Autodesk Inventor part; units mm, degrees
ref_plane "YZ Plane" through (0, 0, 0) normal (1, 0, 0) x (0, 1, 0)
ref_plane "XZ Plane" through (0, 0, 0) normal (0, 1, 0) x (-1, 0, 0)
ref_plane "XY Plane" through (0, 0, 0) normal (0, 0, 1) x (1, 0, 0)
sketch "Sketch1" plane through (0, 0, 0) normal (0, 1, 0) x (-1, 0, 0)
  circle A0 centre (0, 0) radius 63.5
  dimension "d0" = 127
extrude "Extrusion1" add sketch "Sketch1" along normal blind 10
sketch "Sketch2" plane through (0, 0, 0) normal (0, -1, 0) x (1, 0, 0)
  circle A0 centre (0, -44.45) radius 5
  line L0 (0, 0) -> (0, -44.45)
  dimension "d3" = 44.45
  dimension "d4" = 10
extrude "Extrusion2" add sketch "Sketch2" along normal blind 20
sketch "Sketch3" plane through (0, -20, -44.45) normal (0, -1, 0) x (1, 0, 0)
  circle A0 centre (0, 0) radius 5
  arc A1 (0, -7.5) -> (0, 7.5) centre (0, 0) ccw
  line L0 (0, 0) -> (0, -7.5)
  line L1 (0, 0) -> (0, 7.5)
  point P0 (0, 44.45)
  dimension "d7" = 7.5
revolve "Revolution1" add sketch "Sketch3" angle 360 about axis through (0, -20, -44.45) along (0, 0, -1) picked at (1.094, -3.1265) contours A0 L0 L1 | A0 L1 A1 L0
pattern_circular "Circular Pattern1" count 3 over 360 about axis through (0, -10, 0) along (0, 1, 0) of "Extrusion2", "Revolution1"
sketch "Sketch4" plane through (0, 10, 0) normal (0, 1, 0) x (1, 0, 0)
  circle A0 centre (0, 0) radius 10
  dimension "d12" = 20
extrude "Extrusion3" cut sketch "Sketch4" against normal up to surface (10 mm away)
properties part number "pll-base"
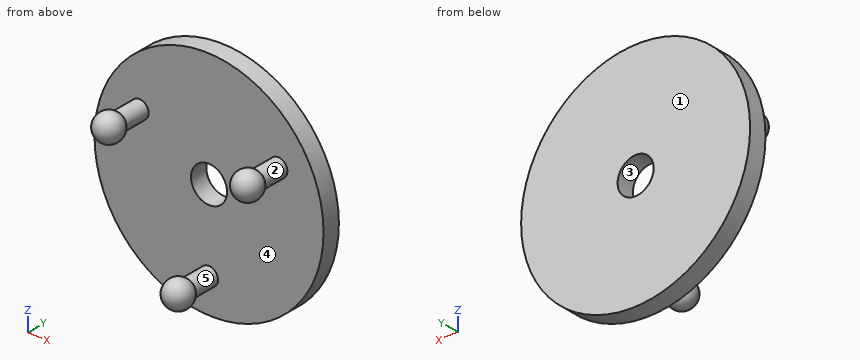
The listing builds one solid part. Answer for the finished solid, in the listing's coordinates (mm). Face numbers are marked on the shaded views. A direction names the side the tool comes from. Coordinates: 2 decimals unless noted, no trailing zeros. Order: outer loops, then holes, each group sorted by start corner. A loop starts at its lowest first (then second) coordinate and runs counter-clockwise, first axis right, second up. Notation, with made-up numbers: M 64.25,14.5 L 81.25,14.5 A20 cw 81.25,41.5 Z; hole C -31.5,84 d6. An arc over 180 degrees is marked long. Use CSV: the item, a comma, the result in double quotes.
Q1. Section D-D (z = -44.45) is taken. Determine the outline of the cut face in (x, y), then the cut area to 3 significant figures.
Here are the results:
outline,"M -45.35,0 L -5,0 L -5,-14.41 A7.5 ccw long 5,-14.41 L 5,0 L 45.35,0 L 45.35,10 L -45.35,10 Z"
area,"1,210 mm2"
Q2. Section B-B (x = 0) is taken. Determine the outline of the cut face in (y, z), then the cut area to 3 significant figures.
Here are the results:
outline,"M -14.41,-49.45 L 0,-49.45 L 0,-63.5 L 10,-63.5 L 10,-10 L 0,-10 L 0,-39.45 L -14.41,-39.45 A7.5 ccw long Z; M 0,10 L 10,10 L 10,63.5 L 0,63.5 Z"
area,"1,380 mm2"
Q3. Section A-A (z = 0) is taken. Determine the outline of the cut face in (x, y), then the cut area to 3 significant figures.
Here are the results:
outline,"M -63.5,0 L -10,0 L -10,10 L -63.5,10 Z; M 10,0 L 63.5,0 L 63.5,10 L 10,10 Z"
area,"1,070 mm2"
Q4. Section C-C (y = 4.5) is taken. Determine the outline of the cut face in (x, z), then the cut area to 3 significant figures.
Here are the results:
outline,"C 0,0 d127; hole C 0,0 d20"
area,"12,400 mm2"
Q5. Determine the mould class of the marked faces 3, 4 and 5 for opening direction Z: pulls with the +Z half, pulls with the -Z half, needs draft (parallel to the pull), parting line crosses it, or undercut.
Here are the results:
face 3,"undercut"
face 4,"needs draft"
face 5,"parting line crosses it"
Q6. Straight lines are drawn through the part: L1, parallel to Z at x = 0, y = 7.5; L2, parallel to Y at x = 29, z = -45.5; L3, parallel to Z at x = -28, y = 1.5. For each, find the intervals that lie inside material, in ascending order.
Here are the results:
L1,"-63.5 to -10, 10 to 63.5"
L2,"0 to 10"
L3,"-56.99 to 56.99"
Q7. A tool of negligible diameter and unlimited length cuts with its end or side. For the marked faces 1 and 2, from which of +Z, -Z, +X, -X, +Y, -Y can it reach the whole face along a straight path? Write none if from no direction.
Here are the results:
face 1,"+Z, -Z, +X, -X, +Y"
face 2,"none"
Q8. Given pin 1 Ø4 at (x, z) = (-30, -37.5) entering from -Y; pin 2 Ø8 at (x, y) = (-1, -23) entering from -Z, each flat-ended and moving along its own axis, determine where each tip first touches the part or whether it passes through.
Here are the results:
pin 1,"y = 0"
pin 2,"z = -51.95"
